Build history of the part. All positions in model axes, mm. Face numbers are marked on the shaded views. A direction names the side the tool comes from. Round coordinates to 2 decimals unless told otherwise and drop trailing zeros. Loops run counter-clockwise (first coordinate to the right, second up) from the corner with the lowest first, then second, coordinate; pieces in that order, holes last. Notation, with made-up numbers: M 9.25,-10 L 60.25,-10 A24 ccw 60.25,22 Z; hole C 50,10.25 d8. An arc over 180 degrees is marked long. One line per item, written item: value.
```python
from build123d import *

# Parameters (mm, degrees)
F0_W      = 34.45
F0_H      = 25.1
F1_DEPTH  = 50.65
F2_T      = -5
F3_R      = 4
F3_R_2    = 0.925
F4_DEPTH  = 25
F5_W      = 31.45
F5_H      = 44.65
F6_DEPTH  = 25.101
F7_R      = 8
F8_R      = 8
F9_R      = 0.925
F10_DEPTH = 50.651


with BuildPart() as f1:
    # F0 (on Top) → F1 (new body)
    with BuildSketch(Plane.XY):
        with Locations((1.9014209259, 12.55)):
            Rectangle(F0_W, F0_H)
    extrude(amount=F1_DEPTH)

    # F2
    f2_openings = [f1.faces().sort_by_distance(p)[0] for p in [
        (-15.323579, 12.55, 25.325),
    ]]
    offset(amount=F2_T, openings=f2_openings)

    # F3 (on face) → F4 (cut)
    with BuildSketch(Plane.YZ.offset(19.1264209259)):
        with Locations((12.55, 25.325)):
            Circle(F3_R)
        with Locations((12.55, 17.475)):
            Circle(F3_R_2)
        with Locations((18.1007882323, 19.7742117677)):
            Circle(F3_R_2)
        with Locations((20.4, 25.325)):
            Circle(F3_R_2)
        with Locations((18.1007882323, 30.8757882323)):
            Circle(F3_R_2)
        with Locations((12.55, 33.175)):
            Circle(F3_R_2)
        with Locations((6.9992117677, 30.8757882323)):
            Circle(F3_R_2)
        with Locations((4.7, 25.325)):
            Circle(F3_R_2)
        with Locations((6.9992117677, 19.7742117677)):
            Circle(F3_R_2)
    extrude(amount=-F4_DEPTH, mode=Mode.SUBTRACT)

    # F5 (on face) → F6 (cut, through all)
    with BuildSketch(Plane(origin=(0, 25.1, 0), x_dir=(-1, 0, 0), z_dir=(0, 1, 0))):
        with Locations((-0.4014209259, 25.325)):
            Rectangle(F5_W, F5_H)
    extrude(amount=-F6_DEPTH, mode=Mode.SUBTRACT)

    # F7
    f7_edges = [f1.edges().sort_by_distance(p)[0] for p in [
        (16.126421, 12.55, 47.65),
        (16.126421, 12.55, 3),
    ]]
    fillet(f7_edges, radius=F7_R)

    # F8
    f8_edges = [f1.edges().sort_by_distance(p)[0] for p in [
        (19.126421, 12.55, 50.65),
        (19.126421, 12.55, 0),
    ]]
    fillet(f8_edges, radius=F8_R)

    # F9 (on face) → F10 (cut, through all)
    with BuildSketch(Plane.XY.offset(50.65)):
        with Locations((-10.2235790741, 19.65)):
            Circle(F9_R)
        with Locations((-10.2235790741, 5.45)):
            Circle(F9_R)
        with BuildLine():
            Line((-4.0485790741, 12.55), (-2.1985790741, 12.55))
            ThreePointArc((-2.1985790741, 12.55), (-3.1235790741, 13.475), (-4.0485790741, 12.55))
        make_face()
        with BuildLine():
            ThreePointArc((-4.0485790741, 12.55), (-3.1235790741, 11.625), (-2.1985790741, 12.55))
            Line((-2.1985790741, 12.55), (-4.0485790741, 12.55))
        make_face()
        with BuildLine():
            ThreePointArc((-10.2235790741, 16.55), (-13.0520061988, 15.3784271247), (-14.2235790741, 12.55))
            Line((-14.2235790741, 12.55), (-6.2235790741, 12.55))
            ThreePointArc((-6.2235790741, 12.55), (-7.3951519493, 15.3784271247), (-10.2235790741, 16.55))
        make_face()
        with BuildLine():
            ThreePointArc((-14.2235790741, 12.55), (-13.0520061988, 9.7215728753), (-10.2235790741, 8.55))
            ThreePointArc((-10.2235790741, 8.55), (-7.3951519493, 9.7215728753), (-6.2235790741, 12.55))
            Line((-6.2235790741, 12.55), (-14.2235790741, 12.55))
        make_face()
        with BuildLine():
            Line((-15.3235790741, 16.55), (-15.3235790741, 12.55))
            Line((-15.3235790741, 12.55), (-14.2235790741, 12.55))
            ThreePointArc((-14.2235790741, 12.55), (-13.0520061988, 15.3784271247), (-10.2235790741, 16.55))
            Line((-10.2235790741, 16.55), (-15.3235790741, 16.55))
        make_face()
        with BuildLine():
            Line((-15.3235790741, 12.55), (-15.3235790741, 8.55))
            Line((-15.3235790741, 8.55), (-10.2235790741, 8.55))
            ThreePointArc((-10.2235790741, 8.55), (-13.0520061988, 9.7215728753), (-14.2235790741, 12.55))
            Line((-14.2235790741, 12.55), (-15.3235790741, 12.55))
        make_face()
    extrude(amount=-F10_DEPTH, mode=Mode.SUBTRACT)


solid = f1.part
```
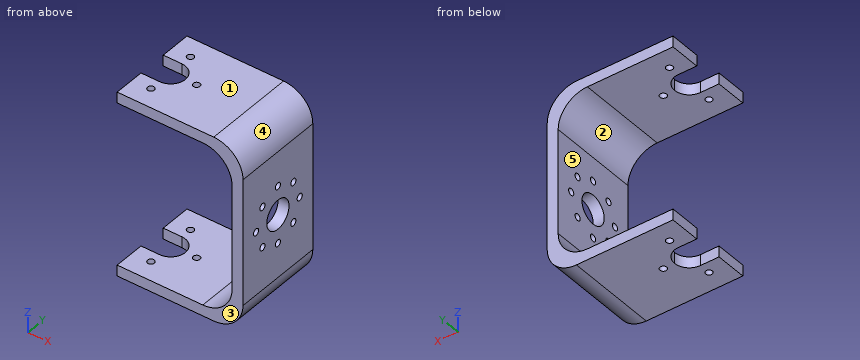
Item 1: Slice it at B-B, the plane z = 15.5. Give the cut face in (x, y).
Check values:
outline: M 16.13,0 L 19.13,0 L 19.13,25.1 L 16.13,25.1 Z
Item 2: Which spindle directions (+Z, -Z, +X, -X, +Y, -Y) get a long thin tool onto all of the face, cutting with end or side? Do the marked faces 1 and 2. Say none if no direction does.
Check values:
face 1: +Z, +X, -X, +Y, -Y
face 2: -X, +Y, -Y
Item 3: Drop flat-ended pins along their axis: P1, Ø2, axis at x = 13, y = 7.5, coming from the -Z side; P2, Ø7.5, axis at y = 10.5, z = 30.5, coming from the -X side. Give the stop position or say it passes through.
Check values:
P1: stops at z = 0.05
P2: stops at x = 16.13
Item 4: Pull direction Z, two halves, no side cores. Call the marked faces 3, 4 and 5: pulls with the +Z half, pulls with the -Z half, needs draft (parallel to the pull), parting line crosses it, or undercut.
Check values:
face 3: needs draft
face 4: pulls with the +Z half
face 5: undercut
Item 5: Slice it at A-A, the plane x = 0. Give the cut face in (y, z), and give its area (3 significant figures).
Check values:
outline: M 0,0 L 25.1,0 L 25.1,3 L 0,3 Z; M 0,47.65 L 25.1,47.65 L 25.1,50.65 L 0,50.65 Z
area: 151 mm2
Item 6: Wall check: line 1 along Z through (x, y) = (-3, 3); line 2 along Z through (x, y) = (17.55, 12.55) (3 decimals); line 3 along Z through (x, y) = (17.3, 12.55) (3 decimals). Give the ranges that are in metal, low to high.
Check values:
line 1: z = 0 to 3, 47.65 to 50.65
line 2: z = 3.232 to 16.55, 18.4 to 21.325, 29.325 to 32.25, 34.1 to 47.418
line 3: z = 2.912 to 16.55, 18.4 to 21.325, 29.325 to 32.25, 34.1 to 47.738
